from build123d import *

# Parameters (mm, degrees)
EXTRUDE_1_DEPTH     = 6
SKETCH_2_R          = 4
CUT_EXTRUDE_1_DEPTH = 6
FILLET_3_R          = 0.3


with BuildPart() as part:
    # 草图1 → 凸台-拉伸1 (new body)
    with BuildSketch(Plane.XY):
        Polygon((0, 7.967433715), (-6.9, 3.983716857), (-6.9, -3.983716857), (0, -7.967433715), (6.9, -3.983716857), (6.9, 3.983716857), align=None)
    extrude(amount=-EXTRUDE_1_DEPTH)

    # 草图2 → 切除-拉伸1 (cut)
    with BuildSketch(Plane.XY):
        Circle(SKETCH_2_R)
    extrude(amount=-CUT_EXTRUDE_1_DEPTH, mode=Mode.SUBTRACT)

    # 草图3 → 切除-旋转2 (revolve, cut)
    with BuildSketch(Plane(origin=(0, 0, 0), x_dir=(0, 0, -1), z_dir=(1, 0, 0))):
        Polygon((0, -7.967433715), (1.05, -7.967433715), (0, -6.917433715), align=None)
        Polygon((6, -7.967433715), (4.95, -7.967433715), (6, -6.917433715), align=None)
    revolve(axis=Axis((0, 0, 0), (0, 0, -1)), mode=Mode.SUBTRACT)

    # 圆角3
    fillet_3_edges = [part.edges().sort_by_distance(p)[0] for p in [
        (-4, 0, -6),
        (-4, 0, 0),
    ]]
    fillet(fillet_3_edges, radius=FILLET_3_R)


solid = part.part
Source: CAD feature listing. Evaluate the final solid. Frame: model axes, mm. Give positions to 0.01 mm unless a question says otherwise; leave off trailing zeros. Write each loop counter-clockwise with the first axis right and the second up, starting at its lowest first coordinate (ties: lowest second). Pieces come first, ordered by that corner, then holes. Notation, with made-up numbers: (-13, -29.5) -> (7, -29.5) arc R17 ccw to (7, -16.5) -> close; hole circle Ø8 at (24, -14.5). An arc over 180 degrees is marked (long way). Return JSON: item names as keys, results as strings. Group by question number.
1. Section B-B, the plane z = -4.25. Output: boundary loops of the cut face in (x, y), then the cut area to 3 significant figures.
2. Mould query, pull axis X, two halves, no side actions, for faces 1 (the face through (0.02, -7.25, -0.33)), 2 (the face through (-0.867, -3.905, -2.962)), 3 (the face through (5, 0, 0)). Classes: +X half, -X half, draft (parallel to the pull), parting line (faces both ways), or undercut.
3. Material intervals for line 1 (X direction, y = 0.25, z = -2.75); line 2 (X direction, y = 0.75, z = -0.75); line 3 (Y direction, x = 4.5, z = -2.25), sorted ascending. Write a range as from..to.
4. Section A-A, the plane y = 0. Output: boundary loops of the cut face in (x, z), then the cut area to 3 significant figures.
5. Section C-C, the plane z = -5.5. Output: boundary loops of the cut face in (x, y).
6. Pin query (flat end, axial travel): pin 1 Ø6 at (x, y) = (-1, -3) entering from -Z; pin 2 Ø2 at (x, z) = (-4.5, -4.5) entering from +Y; pin 3 Ø1.5 at (x, z) = (4.5, -3) entering from -Y; pin 4 Ø2 at (x, z) = (4.5, -5) entering from -Y. Return the tip coordinate at first contact, or that it passes through.
Determined:
{
 "1": {"outline": "(-6.9, -3.98) -> (0, -7.97) -> (6.9, -3.98) -> (6.9, 3.98) -> (0, 7.97) -> (-6.9, 3.98) -> close; hole circle Ø8 at (0, 0)", "area": "115 mm2"},
 "2": {"face 1": "parting line", "face 2": "undercut", "face 3": "draft"},
 "3": {"line 1": "x = -6.9..-3.99, 3.99..6.9", "line 2": "x = -6.9..-3.93, 3.93..6.9", "line 3": "y = -5.37..5.37"},
 "4": {"outline": "(-6.9, -6) -> (-4.3, -6) arc R0.3 ccw to (-4, -5.7) -> (-4, -0.3) arc R0.3 ccw to (-4.3, 0) -> (-6.9, 0) -> close; (4, -5.7) arc R0.3 ccw to (4.3, -6) -> (6.9, -6) -> (6.9, 0) -> (4.3, 0) arc R0.3 ccw to (4, -0.3) -> close", "area": "34.7 mm2"},
 "5": {"outline": "(-6.9, -2.72) arc R7.42 ccw to (-5.81, -4.61) -> (-1.09, -7.34) arc R7.42 ccw to (1.09, -7.34) -> (5.81, -4.61) arc R7.42 ccw to (6.9, -2.72) -> (6.9, 2.72) arc R7.42 ccw to (5.81, 4.61) -> (1.09, 7.34) arc R7.42 ccw to (-1.09, 7.34) -> (-5.81, 4.61) arc R7.42 ccw to (-6.9, 2.72) -> close; hole circle Ø8 at (0, 0)"},
 "6": {"pin 1": "stops at z = -6", "pin 2": "stops at y = 5.95", "pin 3": "stops at y = -5.8", "pin 4": "stops at y = -5.95"}
}
